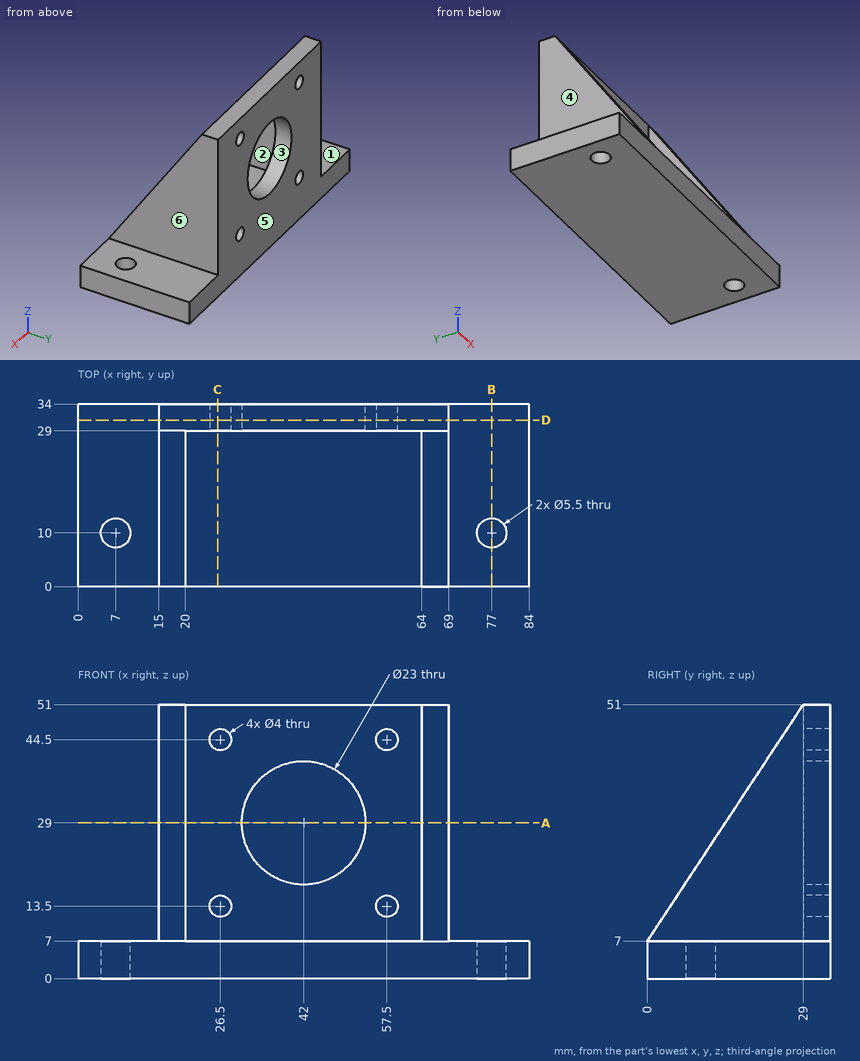
Check sheet for the drawn part. Datum: minimum x, y, z corner. Units: mm. A direction names the side the tool comes from. Coordinates: 2 decimals unless noted, no trailing zeros. Loops run counter-clockwise (first coordinate to the right, second up) from the corner with the lowest first, then second, coordinate; pieces in that order, holes last. Notation, with made-up numbers: (-6.5, -3) -> (19.5, -3) arc R16 ccw to (19.5, 20) -> close; hole circle Ø8 at (3.5, 50). An arc over 180 degrees is marked (long way). Answer in a Markdown table with one row per item.
1. Sectioned sample at A-A, the plane z = 29. Record the boundary of the cut face in (x, y).
Check values:
| item | result |
|---|---|
| outline | (15, 14.5) -> (20, 14.5) -> (20, 29) -> (30.5, 29) -> (30.5, 34) -> (15, 34) -> close; (53.5, 29) -> (64, 29) -> (64, 14.5) -> (69, 14.5) -> (69, 34) -> (53.5, 34) -> close |
2. Access from +Z, -Z, +X, -X, +Y, -Y to the whole of each face (thin tool, end or side, straight path). Record for the marked faces 5 and 6.
Check values:
| item | result |
|---|---|
| face 5 | +Z, -Z, +X, -X, +Y |
| face 6 | +Z, +X, +Y, -Y |
3. Material ranges on line 1 along Z through (x, y) = (26.5, 31); line 2 along X through (y, z) = (32.9, 44.5); line 3 along Y through (x, z) = (77, 3), recorded low to high. Write a range as [from, to].
Check values:
| item | result |
|---|---|
| line 1 | z = [0, 11.5], [15.5, 42.5], [46.5, 51] |
| line 2 | x = [15, 24.5], [28.5, 55.5], [59.5, 69] |
| line 3 | y = [0, 7.25], [12.75, 34] |
4. Go/stop test with flat-tipped pins: pin 1 (14.5 mm diameter, centred on y = 7.5, z = 30.5, fed in from -X); pin 2 (22 mm diameter, centred on x = 33.5, z = 27.5, fed in from -Y); pin 3 (2 mm diameter, centred on y = 26, z = 25.5, fed in from +X); pin 4 (5 mm diameter, centred on x = 26.5, z = 13.5, fed in from +Y). Record where each tip stops, or that it passes through.
Check values:
| item | result |
|---|---|
| pin 1 | stops at x = 15 |
| pin 2 | stops at y = 29 |
| pin 3 | stops at x = 69 |
| pin 4 | stops at y = 34 |
5. Release check for a two-part mould opening along X. For the marked faces 1, 2, 3 and 4 record: released by +X, released by -X, zero draft, split by the parting line, or undercut.
Check values:
| item | result |
|---|---|
| face 1 | zero draft |
| face 2 | undercut |
| face 3 | undercut |
| face 4 | released by -X |
6. Sectioned sample at D-D, the plane y = 31. Record the boundary of the cut face in (x, z).
Check values:
| item | result |
|---|---|
| outline | (0, 0) -> (84, 0) -> (84, 7) -> (69, 7) -> (69, 51) -> (15, 51) -> (15, 7) -> (0, 7) -> close; hole circle Ø4 at (26.5, 13.5); hole circle Ø4 at (26.5, 44.5); hole circle Ø23 at (42, 29); hole circle Ø4 at (57.5, 13.5); hole circle Ø4 at (57.5, 44.5) |
7. Sectioned sample at B-B, the plane x = 77. Record the boundary of the cut face in (y, z), then the cut area to 4 significant figures.
Check values:
| item | result |
|---|---|
| outline | (0, 0) -> (7.25, 0) -> (7.25, 7) -> (0, 7) -> close; (12.75, 0) -> (34, 0) -> (34, 7) -> (12.75, 7) -> close |
| area | 199.5 mm2 |
8. Sectioned sample at C-C, the plane x = 26. Record the boundary of the cut face in (y, z), then the cut area to 3 significant figures.
Check values:
| item | result |
|---|---|
| outline | (0, 0) -> (34, 0) -> (34, 11.56) -> (29, 11.56) -> (29, 7) -> (0, 7) -> close; (29, 15.44) -> (34, 15.44) -> (34, 42.56) -> (29, 42.56) -> close; (29, 46.44) -> (34, 46.44) -> (34, 51) -> (29, 51) -> close |
| area | 419 mm2 |
